from build123d import *

# Parameters (mm, degrees)
BODY_SKETCH_W                        = 10.5
BODY_SKETCH_H                        = 12.5
BODY_DEPTH                           = 9
GEAR_BOX_R                           = 9.5
GEAR_PROFILE_DEPTH                   = 4
SCREWHOLE1_R                         = 1.75
SCREW1_DEPTH                         = 63.032249677
VERRUNDUNG2_R                        = 3
GLIDER_W                             = 9.6
GLIDER_H                             = 61.2
GLIDER_RUT_DEPTH                     = 16
VERRUNDUNG4_R                        = 2
HOLDER_OF_GLIDER_W                   = 4.5
HOLDER_OF_GLIDER_H                   = 8
GLIDER_HOLDER_DEPTH                  = 4.3
VERRUNDUNG5_R                        = 2
VERRUNDUNG6_R                        = 1
VERRUNDUNG7_R                        = 1
PINION_RUT_W                         = 4.5
PINION_RUT_H                         = 72
PINION_RUT_CUT_DEPTH                 = 5
VERRUNDUNG8_R                        = 2
SKETCH_PINION_CHANNEL_W              = 7.3
SKETCH_PINION_CHANNEL_H              = 75
PINION_CHANNEL_DEPTH                 = 6
VERRUNDUNG10_R                       = 1
VERRUNDUNG11_R                       = 1
MOTOR_HOLDER_DEPTH                   = 2
SKIZZE1_R                            = 1
MOTOR_SCREW_DEPTH                    = 10
SCHNITT_LINEAR_AUSTRAGEN2_DEPTH      = 61.991802728
SCHNITT_LINEAR_AUSTRAGEN2_DEPTH_BACK = 2
SKIZZE2_R                            = 2
SCHNITT_LINEAR_AUSTRAGEN3_DEPTH      = 2
VERRUNDUNG12_R                       = 1
VERRUNDUNG13_R                       = 1
LEFT_HOLE_R                          = 1
CENTER_HOLE_LEFT_DEPTH               = 10
ELECTRO_CAGE_DEPTH                   = 16
SKIZZE6_R                            = 1.5
SCHNITT_LINEAR_AUSTRAGEN5_DEPTH      = 18
SKIZZE7_R                            = 1.75
SCHNITT_LINEAR_AUSTRAGEN6_DEPTH      = 18
VERRUNDUNG14_R                       = 3
VERRUNDUNG15_R                       = 5
VERRUNDUNG16_R                       = 1
VERRUNDUNG17_R                       = 1
VERRUNDUNG18_R                       = 1
VERRUNDUNG19_R                       = 1
VERRUNDUNG20_R                       = 1
VERRUNDUNG21_R                       = 3
SKIZZE8_W                            = 2
SKIZZE8_H                            = 4
SCHNITT_LINEAR_AUSTRAGEN7_DEPTH      = 2
VERRUNDUNG22_R                       = 0.5


# Some blends are built 0.0001 mm under size
with BuildPart() as part:
    # body-sketch → body (new, symmetric)
    with BuildSketch(Plane.XY):
        Polygon((-32, 50), (0, 50), (0, -22), (-17, -22), (-17, 0), (-32, 0), align=None)
        with Locations((-20.75, 36.75)):
            Rectangle(BODY_SKETCH_W, BODY_SKETCH_H, mode=Mode.SUBTRACT)
    extrude(amount=BODY_DEPTH, both=True)

    # gear_box → gear_profile (cut)
    with BuildSketch(Plane.XY.offset(9)):
        with Locations((-20.75, 36.75)):
            Circle(GEAR_BOX_R)
    extrude(amount=-GEAR_PROFILE_DEPTH, mode=Mode.SUBTRACT)

    # screwhole1 → screw1 (cut, through all)
    with BuildSketch(Plane.XY.offset(9)):
        with Locations((-28.5, 46.5)):
            Circle(SCREWHOLE1_R)
        with Locations((-3.677178533, 46.5)):
            Circle(SCREWHOLE1_R)
        with Locations((-2.8, -19.2)):
            Circle(SCREWHOLE1_R)
    extrude(amount=-SCREW1_DEPTH, mode=Mode.SUBTRACT)

    # Verrundung2
    verrundung2_edges = [part.edges().sort_by_distance(p)[0] for p in [
        (-32, 50, 0),
        (0, 50, 0),
    ]]
    fillet(verrundung2_edges, radius=VERRUNDUNG2_R)

    # glider → glider_rut (cut)
    with BuildSketch(Plane.XY.offset(9)):
        with Locations((-8.2, 13.3)):
            Rectangle(GLIDER_W, GLIDER_H)
    extrude(amount=-GLIDER_RUT_DEPTH, mode=Mode.SUBTRACT)

    # Verrundung4
    verrundung4_edges = [part.edges().sort_by_distance(p)[0] for p in [
        (-13, 31.255684756, 7),
    ]]
    fillet(verrundung4_edges, radius=VERRUNDUNG4_R)

    # holder of glider → glider-holder (add)
    with BuildSketch(Plane.XY.offset(-7)):
        with Locations((-8.95, 26.8)):
            Rectangle(HOLDER_OF_GLIDER_W, HOLDER_OF_GLIDER_H)
        with Locations((-7.45, -1.3)):
            Rectangle(HOLDER_OF_GLIDER_W, HOLDER_OF_GLIDER_H)
    extrude(amount=GLIDER_HOLDER_DEPTH)

    # Verrundung5
    verrundung5_edges = [part.edges().sort_by_distance(p)[0] for p in [
        (-6.7, 22.8, -4.85),
        (-6.7, 30.8, -4.85),
        (-11.2, 30.8, -4.85),
        (-11.2, 22.8, -4.85),
        (-5.2, -5.3, -4.85),
        (-5.2, 2.7, -4.85),
        (-9.7, 2.7, -4.85),
        (-9.7, -5.3, -4.85),
    ]]
    fillet(verrundung5_edges, radius=VERRUNDUNG5_R)

    # Verrundung6
    verrundung6_edges = [part.edges().sort_by_distance(p)[0] for p in [
        (-11.2, 26.8, -7),
        (-8.95, 30.8, -7),
        (-6.7, 26.8, -7),
        (-8.95, 22.8, -7),
        (-10.614213562, 30.214213562, -7),
        (-7.285786438, 30.214213562, -7),
        (-7.285786438, 23.385786438, -7),
        (-10.614213562, 23.385786438, -7),
    ]]
    fillet(verrundung6_edges, radius=VERRUNDUNG6_R)

    # Verrundung7
    verrundung7_edges = [part.edges().sort_by_distance(p)[0] for p in [
        (-7.45, -5.3, -7),
        (-9.7, -1.3, -7),
        (-5.2, -1.3, -7),
        (-7.45, 2.7, -7),
        (-9.114213562, -4.714213562, -7),
        (-5.785786438, -4.714213562, -7),
        (-5.785786438, 2.114213562, -7),
        (-9.114213562, 2.114213562, -7),
    ]]
    fillet(verrundung7_edges, radius=VERRUNDUNG7_R)

    # Pinion rut → pinion rut cut (cut)
    with BuildSketch(Plane.XY.offset(9)):
        with Locations((-9.5, 14)):
            Rectangle(PINION_RUT_W, PINION_RUT_H)
    extrude(amount=-PINION_RUT_CUT_DEPTH, mode=Mode.SUBTRACT)

    # Verrundung8
    # the kernel refuses this fillet: 2 mm, written as the material it takes off along each edge
    with BuildSketch(Plane(origin=(-13, 42.244315244, 5), x_dir=(0, 1, 0), z_dir=(0, 0, 1))) as verrundung8_piece_1:
        with BuildLine():
            CenterArc((3.548666653, 0.645460718), VERRUNDUNG8_R, 141.845362101, 56.982763935)
            Line((1.975974149, 1.881032767), (1.944520299, 1.905744208))
            ThreePointArc((1.944520299, 1.905744208), (1.028281735, 0.89818793), (-0.023133959, 0.032631579))
            Line((-0.023133959, 0.032631579), (0, -0.04))
            ThreePointArc((0, -0.04), (0.827842378, -0.04), (1.617825118, -0.012909214))
            Line((1.617825118, -0.012909214), (1.655684756, 0))
        make_face()
    extrude(amount=10.820354696, mode=Mode.SUBTRACT)

    # sketch pinion channel → pinion channel (cut)
    with BuildSketch(Plane.XY.offset(9)):
        with Locations((-10.9, 12.5)):
            Rectangle(SKETCH_PINION_CHANNEL_W, SKETCH_PINION_CHANNEL_H)
    extrude(amount=-PINION_CHANNEL_DEPTH, mode=Mode.SUBTRACT)

    # Verrundung10
    verrundung10_edges = [part.edges().sort_by_distance(p)[0] for p in [
        (-7.25, -17.3, 6),
        (-7.25, 50, 6),
        (-14.55, 50, 6),
    ]]
    fillet(verrundung10_edges, radius=VERRUNDUNG10_R)

    # Verrundung11
    verrundung11_edges = [part.edges().sort_by_distance(p)[0] for p in [
        (-10.125, 43.9, 3),
        (-9.625, -17.3, 3),
        (-10.9, 50, 3),
    ]]
    fillet(verrundung11_edges, radius=VERRUNDUNG11_R)

    # motor-holder 2 → motor -holder (cut)
    with BuildSketch(Plane.XY.offset(5)):
        Polygon((-14.33941219, 43.85), (-14.33941219, 29.65), (-17.83941219, 29.65), (-17.83941219, 27.95), (-23.83941219, 27.95), (-23.83941219, 29.65), (-26.63941219, 29.65), (-26.63941219, 43.85), (-23.83941219, 43.85), (-23.83941219, 45.55), (-17.83941219, 45.55), (-17.83941219, 43.85), align=None)
    extrude(amount=-MOTOR_HOLDER_DEPTH, mode=Mode.SUBTRACT)

    # Skizze1 → motor-screw (cut)
    with BuildSketch(Plane.XY.offset(3)):
        with Locations((-20.83941219, 28.75)):
            Circle(SKIZZE1_R)
        with Locations((-20.83941219, 44.75)):
            Circle(SKIZZE1_R)
    extrude(amount=-MOTOR_SCREW_DEPTH, mode=Mode.SUBTRACT)

    # Skizze2 → Schnitt-Linear austragen2 (cut, two sides: drawn at the far end of the back side and taken through both)
    with BuildSketch(Plane.XY.offset(5).offset(-SCHNITT_LINEAR_AUSTRAGEN2_DEPTH_BACK)):
        with Locations((-20.83941219, 44.75)):
            Circle(SKIZZE2_R)
        with Locations((-20.83941219, 28.75)):
            Circle(SKIZZE2_R)
    extrude(amount=SCHNITT_LINEAR_AUSTRAGEN2_DEPTH + SCHNITT_LINEAR_AUSTRAGEN2_DEPTH_BACK, mode=Mode.SUBTRACT)

    # Skizze3 → Schnitt-Linear austragen3 (cut)
    with BuildSketch(Plane.XY.offset(5)):
        with BuildLine():
            Line((-26.63941219, 40.25), (-26.63941219, 33.25))
            ThreePointArc((-26.63941219, 33.25), (-30.13941219, 36.75), (-26.63941219, 40.25))
        make_face()
    extrude(amount=-SCHNITT_LINEAR_AUSTRAGEN3_DEPTH, mode=Mode.SUBTRACT)

    # Verrundung12
    verrundung12_edges = [part.edges().sort_by_distance(p)[0] for p in [
        (-14.55, 29.65, 4),
        (-14.55, 43.85, 4),
    ]]
    fillet(verrundung12_edges, radius=VERRUNDUNG12_R)

    # Verrundung13
    verrundung13_edges = [part.edges().sort_by_distance(p)[0] for p in [
        (-26.63941219, 33.25, 4),
        (-26.63941219, 40.25, 4),
    ]]
    fillet(verrundung13_edges, radius=VERRUNDUNG13_R)

    # left hole → center-hole-left (cut)
    with BuildSketch(Plane.XY.offset(3)):
        with Locations((-28, 36.75)):
            Circle(LEFT_HOLE_R)
    extrude(amount=-CENTER_HOLE_LEFT_DEPTH, mode=Mode.SUBTRACT)

    # cage → electro-cage (cut)
    with BuildSketch(Plane.XY.offset(9)):
        Polygon((-30, 25.412090366), (-30, 7.737950254), (-24.052522804, 7.737950254), (-24.052522804, 2), (-16.55, 2), (-16.55, 7.140007769), (-7.441971484, 7.140007769), (-7.441971484, 18.806564473), (-16.55, 18.806564473), (-16.55, 25.412090366), align=None)
    extrude(amount=-ELECTRO_CAGE_DEPTH, mode=Mode.SUBTRACT)

    # Skizze6 → Schnitt-Linear austragen5 (cut)
    with BuildSketch(Plane.XY.offset(9)):
        with Locations((-25.237300627, 25.412090366)):
            Circle(SKIZZE6_R)
    extrude(amount=-SCHNITT_LINEAR_AUSTRAGEN5_DEPTH, mode=Mode.SUBTRACT)

    # Skizze7 → Schnitt-Linear austragen6 (cut)
    with BuildSketch(Plane.XY.offset(9)):
        with Locations((-28.5, 3.5)):
            Circle(SKIZZE7_R)
    extrude(amount=-SCHNITT_LINEAR_AUSTRAGEN6_DEPTH, mode=Mode.SUBTRACT)

    # Verrundung14
    verrundung14_edges = [part.edges().sort_by_distance(p)[0] for p in [
        (-32, 0, 0),
    ]]
    fillet(verrundung14_edges, radius=VERRUNDUNG14_R)

    # Verrundung15
    verrundung15_edges = [part.edges().sort_by_distance(p)[0] for p in [
        (-24.052522804, 7.737950254, 1),
    ]]
    fillet(verrundung15_edges, radius=VERRUNDUNG15_R)

    # Verrundung16
    verrundung16_edges = [part.edges().sort_by_distance(p)[0] for p in [
        (-16.55, 18.806564473, 1),
    ]]
    fillet(verrundung16_edges, radius=VERRUNDUNG16_R)

    # Verrundung17
    verrundung17_edges = [part.edges().sort_by_distance(p)[0] for p in [
        (-16.55, 7.140007769, 1),
    ]]
    fillet(verrundung17_edges, radius=VERRUNDUNG17_R)

    # Verrundung18
    # the kernel refuses this fillet: 1 mm, written as the material it takes off along each edge
    with BuildSketch(Plane(origin=(-23.737300627, 25.412090366, 10.978219619), x_dir=(-0.20430964368921942, 0.9789063129307034, 0), z_dir=(0, 0, -1))) as verrundung18_piece_1:
        with BuildLine():
            CenterArc((0.817238575, 0.978906313), VERRUNDUNG18_R, 191.789089239, 66.421821522)
            Line((-0.161667738, 0.774596669), (0, 0))
            ThreePointArc((0, 0), (0.306464466, 0.031640531), (0.612928931, 0))
        make_face()
    extrude(amount=17.978219619, mode=Mode.SUBTRACT)

    # Verrundung19
    verrundung19_edges = [part.edges().sort_by_distance(p)[0] for p in [
        (-13, 18.806564473, -2),
        (-13, 7.140007769, -2),
        (-14.55, 7.140007769, 6),
        (-14.55, 18.806564473, 6),
    ]]
    fillet(verrundung19_edges, radius=VERRUNDUNG19_R - 0.0001)  # a hair under: the kernel refuses the full size

    # Verrundung20
    verrundung20_edges = [part.edges().sort_by_distance(p)[0] for p in [
        (-26.737300627, 25.412090366, 1),
    ]]
    fillet(verrundung20_edges, radius=VERRUNDUNG20_R)

    # Verrundung21
    verrundung21_edges = [part.edges().sort_by_distance(p)[0] for p in [
        (-17, -22, 0),
        (0, -22, 0),
    ]]
    fillet(verrundung21_edges, radius=VERRUNDUNG21_R)

    # Skizze8 → Schnitt-Linear austragen7 (cut)
    with BuildSketch(Plane.XY.offset(9)):
        with Locations((-31, 14)):
            Rectangle(SKIZZE8_W, SKIZZE8_H)
    extrude(amount=-SCHNITT_LINEAR_AUSTRAGEN7_DEPTH, mode=Mode.SUBTRACT)

    # Verrundung22
    verrundung22_edges = [part.edges().sort_by_distance(p)[0] for p in [
        (-31, 16, 7),
        (-31, 12, 7),
    ]]
    fillet(verrundung22_edges, radius=VERRUNDUNG22_R)


solid = part.part
Verification items for the finished model (mm, model axes). A direction names the side the tool comes from. Give positions to 0.01 mm unless a question says otherwise; leave off trailing zeros. Loops run counter-clockwise (first coordinate to the right, second up) from the corner with the lowest first, then second, coordinate; pieces in that order, holes last. Notation, with made-up numbers: (87, 38) - (117, 38) arc R13 cw to (117, 47) - close; hole circle Ø3 at (32.25, -0.75). An arc over 180 degrees is marked (long way). Write each question's results on one line, items separated by ' | '.
1) Depth check by flat-ended pin: P1, Ø1, axis at x = -25, z = 4, coming from the -Y side; P2, Ø1.3, axis at x = -8.5, y = 26, coming from the +Z side; P3, Ø0.8, axis at x = -31, z = 8, coming from the +Y side. Enter the tip coordinate at first touch or a pass-through.
Solution:
P1: y = 0 | P2: z = -2.7 | P3: y = 49.54
2) Sectioned sample at A-A on y = -8.5. Record the boundary of the cut face in (x, z), plus the area to 3 significant figures.
Solution:
outline: (-17, -9) - (0, -9) - (0, 9) - (-3.4, 9) - (-3.4, -7) - (-13, -7) - (-13, 3) - (-14.55, 3) - (-14.55, 9) - (-17, 9) - close | area: 143 mm2
3) Sectioned sample at C-C on y = 34. Record the boundary of the cut face in (x, z).
Solution:
outline: (-32, -9) - (-26, -9) - (-26, 3) - (-28.8, 3) - (-28.8, 5) - (-29.84, 5) - (-29.84, 9) - (-32, 9) - close; (-15.5, -9) - (0, -9) - (0, 9) - (-3.4, 9) - (-3.4, -7) - (-13, -7) - (-13, 3) - (-15.5, 3) - close
4) Mould release check, pull along Y, two halves, no side actions. Record for faces 4 (the flat face through (-2, 15, 9)), 5 (the cylindrical face through (-7.3, 23.37, -4.33)), 6 (the flat face through (-7, -17.3, -1)), 7 (the flat face through (-16, 50, 0)): pulls with the +Y half, pulls with the -Y half, needs draft (parallel to the pull), parting line crosses it, or undercut.
Solution:
face 4: needs draft | face 5: undercut | face 6: undercut | face 7: pulls with the +Y half
5) Sectioned sample at B-B on z = -8. Record the boundary of the cut face in (x, y).
Solution:
outline: (-32, 3) arc R3 ccw to (-29, 0) - (-17, 0) - (-17, -19) arc R3 ccw to (-14, -22) - (-3, -22) arc R3 ccw to (0, -19) - (0, 47) arc R3 ccw to (-3, 50) - (-29, 50) arc R3 ccw to (-32, 47) - close; hole circle Ø3.5 at (-28.5, 3.5); hole circle Ø3.5 at (-28.5, 46.5); hole circle Ø3 at (-25.24, 25.41); hole (-26, 30.5) - (-15.5, 30.5) - (-15.5, 43) - (-26, 43) - close; hole circle Ø3.5 at (-3.68, 46.5); hole circle Ø3.5 at (-2.8, -19.2)
6) Material ranges on L1, parallel to X at y = 21, z = 1.25; L2, parallel to Y at x = -21, z = 0; L3, parallel to Y at x = -23, z = -6, recorded low to high. Write a range as from..to.
Solution:
L1: -32..-30, -16.55..-13, -3.4..0 | L2: 0..2, 25.41..27.76, 29.74..30.5, 43..43.76, 45.74..50 | L3: 0..2, 25.41..30.5, 43..50
7) Tool access check on faces 1 (the flat face through (-14.55, 47, 6)), 2 (the flat face through (-6.7, 27, -4)), 3 (the flat face through (-31, 12, 8)). Record the directions out of +Z, -Z, +X, -X, +Y, -Y that give a thin tool (end or side, any length) a straight path to the whole face; none if there is none.
Solution:
face 1: +Z, +Y, -Y | face 2: +Z | face 3: +Z, -X
